Read the model definition and answer for the solid it produces. Units are mm, in the model's axes. A direction names the side the tool comes from. Coordinates: 2 decimals unless noted, no trailing zeros. Write each loop counter-clockwise with the first axis right and the second up, starting at its lowest first coordinate (ties: lowest second). Pieces come first, ordered by that corner, then holes. Notation, with made-up numbers: (-11.5, 48) -> (35.5, 48) arc R25 ccw to (35.5, 80) -> close; hole circle Ø10 at (-20, 20). An arc over 180 degrees is marked (long way). Return JSON: item names as keys, results as strings.
from build123d import *

# Parameters (mm, degrees)
SKETCH1_R           = 15
BOSS_EXTRUDE1_DEPTH = 15
SKETCH2_R           = 10
BOSS_EXTRUDE2_DEPTH = 20
SKETCH3_R           = 10
BOSS_EXTRUDE3_DEPTH = 20


with BuildPart() as part:
    # Sketch1 → Boss-Extrude1 (new body, symmetric)
    with BuildSketch(Plane.XY):
        Circle(SKETCH1_R)
    extrude(amount=BOSS_EXTRUDE1_DEPTH, both=True)

    # Sketch2 → Boss-Extrude2 (add)
    with BuildSketch(Plane.XY.offset(15)):
        Circle(SKETCH2_R)
    extrude(amount=BOSS_EXTRUDE2_DEPTH)

    # Sketch3 → Boss-Extrude3 (add)
    with BuildSketch(Plane(origin=(0, 0, -15), x_dir=(-1, 0, 0), z_dir=(0, 0, -1))):
        Circle(SKETCH3_R)
    extrude(amount=BOSS_EXTRUDE3_DEPTH)


solid = part.part
1. The part is cut by section D-D (z = -4). Determine the outline of the cut face in (x, y).
Taken from the geometry:
{"outline": "circle Ø30 at (0, 0)"}
2. Flat-ended cylindrical pins translate along their axes: pin 1 Ø5 at (x, y) = (-10, 10.5) entering from +Z; pin 2 Ø3 at (y, z) = (-9, -28) entering from +X; pin 3 Ø10 at (x, z) = (-1.5, 14.5) entering from +Y; pin 4 Ø4 at (x, z) = (4.5, -26) entering from -Y. Find the tip coordinate at first contact, or state that the pin passes through.
Taken from the geometry:
{"pin 1": "stops at z = 15", "pin 2": "stops at x = 6.61", "pin 3": "stops at y = 15", "pin 4": "stops at y = -9.68"}
3. The part is cut by section A-A (y = 0). Determine the outline of the cut face in (x, z).
Taken from the geometry:
{"outline": "(-15, -15) -> (-10, -15) -> (-10, -35) -> (10, -35) -> (10, -15) -> (15, -15) -> (15, 15) -> (10, 15) -> (10, 35) -> (-10, 35) -> (-10, 15) -> (-15, 15) -> close"}
4. Consider L1, parallel to Z at x = 13.5, y = -2; L2, parallel to X at y = 6, z = -25; L3, parallel to Y at x = 9, z = 16.5. Determine where each line is inside the solid, lowest interval first.
Taken from the geometry:
{"L1": "z = -15 to 15", "L2": "x = -8 to 8", "L3": "y = -4.36 to 4.36"}
5. The part is cut by section C-C (z = 24). Determine the outline of the cut face in (x, y), then the cut area to 3 significant figures.
Taken from the geometry:
{"outline": "circle Ø20 at (0, 0)", "area": "314 mm2"}
6. A tool of negligible diameter and unlimited length cuts with its end or side. For faces 1 (the face through (2.17, -9.76, -24.86)), 2 (the face through (0, 0, -35)), 3 (the face through (3, -10, 15)), from which of +Z, -Z, +X, -X, +Y, -Y can it reach the whole face along a straight path? Write none if from no direction.
Taken from the geometry:
{"face 1": "-Z", "face 2": "-Z, +X, -X, +Y, -Y", "face 3": "+Z"}
